Autodesk Inventor part; units mm, degrees
ref_plane "YZ Plane" through (0, 0, 0) normal (1, 0, 0) x (0, 1, 0)
ref_plane "XZ Plane" through (0, 0, 0) normal (0, 1, 0) x (-1, 0, 0)
ref_plane "XY Plane" through (0, 0, 0) normal (0, 0, 1) x (1, 0, 0)
sketch "Sketch1" plane through (0, 0, 0) normal (0, 0, 1) x (1, 0, 0)
  line L0 (-11.1125, 0) -> (11.1125, 0)
  line L1 (0, -15.5575) -> (0, 15.5575)
  line L2 (-7.9375, 11.1125) -> (7.9375, 11.1125)
  line L3 (7.9375, 11.1125) -> (7.9375, -11.1125)
  line L4 (7.9375, -11.1125) -> (-7.9375, -11.1125)
  line L5 (-7.9375, -11.1125) -> (-7.9375, 11.1125)
  point P0 (0, 0)
  point P1 (-7.9375, 0)
  point P2 (0, 11.1125)
  dimension "d0" = 15.875
  dimension "d1" = 22.225
extrude "Extrusion1" add sketch "Sketch1" along normal blind 4.7625
sketch "Sketch2" plane through (0, 0, 4.7625) normal (0, 0, 1) x (1, 0, 0)
  line L0 (4.3656, 4.7625) -> (4.3656, -4.7625)
  line L1 (-4.3656, -4.7625) -> (-4.3656, 4.7625)
  line L2 (-1.1906, 4.7625) -> (-1.1906, -4.7625)
  line L3 (1.1906, 4.7625) -> (1.1906, -4.7625)
  line L4 (-4.3656, 4.7625) -> (-1.1906, 4.7625)
  line L5 (1.1906, 4.7625) -> (4.3656, 4.7625)
  line L6 (4.3656, -4.7625) -> (1.1906, -4.7625)
  line L7 (-1.1906, -4.7625) -> (-4.3656, -4.7625)
  line L8 (1.1906, 4.7625) -> (-1.1906, 4.7625) construction
  line L9 (-1.1906, -4.7625) -> (1.1906, -4.7625) construction
  point P0 (0, 0)
  point P1 (-4.3656, 0)
  point P2 (0, 6.35)
  point P3 (0, 4.7625)
  dimension "d5" = 9.525
  dimension "d10" = 2.3813
  dimension "d11" = 3.175
extrude "Extrusion4" add sketch "Sketch2" along normal blind 12.7
sketch "Sketch4" plane through (4.3656, -4.7625, 4.7625) normal (1, 0, 0) x (0, 0, -1)
  line L0 (-12.7, 9.525) -> (-12.7, 0)
  line L1 (0, 0) -> (-12.7, 0)
  line L2 (0, 9.525) -> (0, 0)
  line L3 (0, 9.525) -> (-12.7, 9.525)
  arc A0 (-7.9375, 9.525) -> (-7.9375, 0) centre (-7.9375, 4.7625) ccw
  point P0 (4.7625, 4.7625)
extrude "Extrusion5" cut sketch "Sketch4" against normal through all contours L3 A0 L0 | A0 L1 L0
properties part number "piston mount bracket"
Here's how the part is built. I have some questions about the finished solid (model axes, mm). A direction names the side the tool comes from. Round coordinates to 2 decimals unless told otherwise and drop trailing zeros. Loops run counter-clockwise (first coordinate to the right, second up) from the corner with the lowest first, then second, coordinate; pieces in that order, holes last. Notation, with made-up numbers: (14.5, -29.5) -> (39.5, -29.5) arc R27 cw to (39.5, 0.5) -> close; hole circle Ø9 at (-6, -5). An arc over 180 degrees is marked (long way). Answer as CSV lines item,"result". Start each with the question number.
1. Imagine slicing it at C-C on y = 0. Write out the boundary of the cut face in (x, z), plus the area to 3 significant figures.
2. For faces 1 (the face through (4.366, 0, 11)), 2 (the face through (1.191, 0, 11)), 3 (the face through (-3, 4.762, 9)), 4 (the face through (-4.366, 0, 11)), 5 (the face through (3, -4.762, 9)), which set-ups out of +Z, -Z, +X, -X, +Y, -Y let a thin tool reach every point of the face, with its end or its side?
3. Imagine slicing it at A-A on z = 10.75. Write out the boundary of the cut face in (x, y), plus the area to 3 significant figures.
4. Imagine slicing it at D-D on z = 16. Write out the boundary of the cut face in (x, y).
5. If we mould it in two halves opening along X, with no side actions, what happens to faces 6 (the face through (-7.938, 0, 2)), 7 (the face through (-1.191, 0, 11)), 8 (the face through (-3, -4.762, 9))? For each: pulls with the +X half, pulls with the -X half, needs draft (parallel to the pull), parting line crosses it, or undercut.
6. Imagine slicing it at B-B on x = -1.5. Write out the boundary of the cut face in (y, z) (1 decimal), plus the area to 3 significant figures.
7. I'm going to push flat-ended pins straight in: P1, Ø8, axis at y = -6, z = 10.5, coming from the -X side; P2, Ø1, axis at x = 2, z = 9.5, coming from the -Y side; P3, Ø5, axis at y = -0.5, z = 10, coming from the +X side; P4, Ø5, axis at x = 1, y = -1.5, coming from the +Z side. Where does each tip first touch, or does it pass through?
8. I need wall thicknesses on probe 1 along X at (y, z) = (0.5, 9.5); probe 2 along Z at (x, y) = (6.5, -4); probe 3 along Y at (x, z) = (4.25, 10.5). Which ranges of each line are inside material? Lowest first, please. Write a range as from..to.
Solution:
1,outline,"(-7.94, 0) -> (7.94, 0) -> (7.94, 4.76) -> (4.37, 4.76) -> (4.37, 17.46) -> (1.19, 17.46) -> (1.19, 4.76) -> (-1.19, 4.76) -> (-1.19, 17.46) -> (-4.37, 17.46) -> (-4.37, 4.76) -> (-7.94, 4.76) -> close"
1,area,"156 mm²"
2,face 1,"+Z, +X, +Y, -Y"
2,face 2,"+Z, +Y, -Y"
2,face 3,"+Z, +X, -X, +Y"
2,face 4,"+Z, -X, +Y, -Y"
2,face 5,"+Z, +X, -X, -Y"
3,outline,"(-4.37, -4.76) -> (-1.19, -4.76) -> (-1.19, 4.76) -> (-4.37, 4.76) -> close; (1.19, -4.76) -> (4.37, -4.76) -> (4.37, 4.76) -> (1.19, 4.76) -> close"
3,area,"60.5 mm²"
4,outline,"(-4.37, -3.43) -> (-1.19, -3.43) -> (-1.19, 3.43) -> (-4.37, 3.43) -> close; (1.19, -3.43) -> (4.37, -3.43) -> (4.37, 3.43) -> (1.19, 3.43) -> close"
5,face 6,"pulls with the -X half"
5,face 7,"undercut"
5,face 8,"needs draft"
6,outline,"(-11.1, 0) -> (11.1, 0) -> (11.1, 4.8) -> (4.8, 4.8) -> (4.8, 12.7) arc R4.8 ccw to (-4.8, 12.7) -> (-4.8, 4.8) -> (-11.1, 4.8) -> close"
6,area,"217 mm²"
7,P1,"x = -4.37"
7,P2,"y = -4.76"
7,P3,"x = 4.37"
7,P4,"z = 17.46"
8,probe 1,"-4.37..-1.19, 1.19..4.37"
8,probe 2,"0..4.76"
8,probe 3,"-4.76..4.76"
